The model under review builds one solid part; all positions refer to its coordinate system, in mm. Coordinates: 2 decimals unless noted, no trailing zeros. Loops run counter-clockwise (first coordinate to the right, second up) from the corner with the lowest first, then second, coordinate; pieces in that order, holes last. Notation, with made-up numbers: M -5.5,62 L 23.5,62 A20 cw 23.5,93 Z; hole C 86,50 d7. An arc over 180 degrees is marked long. Write item = value, one per line. Start each with the question number.
Q1. Clearance check with flat-ended pins moving along their axes: pin 1 Ø2.5 at (x, y) = (0, 0) entering from -Z; pin 2 Ø1 at (x, z) = (1, 0.5) entering from +Y. State where each tip first meets the part, or that it passes through.
Q2. We need section A-A on x = 0. Give the boundary of the cut face in (y, z).
Q3. Mouldability with a two-part tool opening along X and no side actions: class faces 1 (the face through (0.05, -2.25, -0.03)), 2 (the face through (-0.325, 33.714, -0.028)), 3 (the face through (0, 16, -2)), 4 (the face through (-1.5, -0.07, -0.03)) as released by +X, released by -X, zero draft, split by the parting line, or undercut.
Q4. We need section B-B on z = -0.4. Give the boundary of the cut face in (x, y).
Q5. Wall thickness on probe 1 along Y at (x, z) = (0, -0.2); probe 2 along Y at (x, z) = (0.9, -1.4); probe 3 along X at (y, z) = (33, -1.05): over which ranges is each line inside the solid? List them lowest first.
Autodesk Inventor part; units mm, degrees
ref_plane "YZ Plane" through (0, 0, 0) normal (1, 0, 0) x (0, 1, 0)
ref_plane "XZ Plane" through (0, 0, 0) normal (0, 1, 0) x (-1, 0, 0)
ref_plane "XY Plane" through (0, 0, 0) normal (0, 0, 1) x (1, 0, 0)
sketch "Sketch1" plane through (0, 0, 0) normal (0, 0, 1) x (1, 0, 0)
  line L0 (0, 0) -> (0, 32.25) construction
  line L1 (2.25, 0) -> (2.25, 32.25)
  line L2 (-2.25, 32.25) -> (-2.25, 0)
  arc A0 (-2.25, 0) -> (2.25, 0) centre (0, 0) ccw
  arc A1 (2.25, 32.25) -> (-2.25, 32.25) centre (0, 32.25) ccw
  circle A2 centre (0, 0) radius 1.5
  circle A3 centre (0, 32.25) radius 1.5
  point P0 (0, 16.125)
  dimension "d0" = 32.25
  dimension "d1" = 4.5
  dimension "d2" = 3
  dimension "d3" = 3
extrude "Extrusion1" add sketch "Sketch1" along normal mid plane 4
properties part number "un"
Returned:
q1.pin_1 = through
q1.pin_2 = 34.44
q2.outline = M -2.25,-2 L -1.5,-2 L -1.5,2 L -2.25,2 Z; M 1.5,-2 L 30.75,-2 L 30.75,2 L 1.5,2 Z; M 33.75,-2 L 34.5,-2 L 34.5,2 L 33.75,2 Z
q3.face_1 = split by the parting line
q3.face_2 = undercut
q3.face_3 = zero draft
q3.face_4 = undercut
q4.outline = M -2.25,0 A2.25 ccw 2.25,0 L 2.25,32.25 A2.25 ccw -2.25,32.25 Z; hole C 0,0 d3; hole C 0,32.25 d3
q5.probe_1 = -2.25 to -1.5, 1.5 to 30.75, 33.75 to 34.5
q5.probe_2 = -2.06 to -1.2, 1.2 to 31.05, 33.45 to 34.31
q5.probe_3 = -2.12 to -1.3, 1.3 to 2.12
